from build123d import *

# Parameters (mm, degrees)
SKETCH1_R           = 3
BOSS_EXTRUDE1_DEPTH = 1.59


with BuildPart() as part:
    # Sketch1 → Boss-Extrude1 (new body)
    with BuildSketch(Plane.XY):
        with BuildLine():
            ThreePointArc((-5.900608413, 13.97128969), (-4.905988344, 14.048559559), (-4.072428842, 14.59666381))
            ThreePointArc((-4.072428842, 14.59666381), (3.290759997, 15.306914867), (4.701099283, 8.045238095))
            ThreePointArc((4.701099283, 8.045238095), (3.974825904, 5.45), (4.701099283, 2.854761905))
            ThreePointArc((4.701099283, 2.854761905), (0, -5.5), (-4.701099283, 2.854761905))
            ThreePointArc((-4.701099283, 2.854761905), (-3.974825904, 5.45), (-4.701099283, 8.045238095))
            ThreePointArc((-4.701099283, 8.045238095), (-4.911398404, 8.424486778), (-5.091164818, 8.819124992))
            ThreePointArc((-5.091164818, 8.819124992), (-5.686991836, 9.619268653), (-6.595201124, 10.032058678))
            Line((-6.595201124, 10.032058678), (-25.459894057, 13.358413024))
            Line((-25.459894057, 13.358413024), (-24.765301346, 17.297644037))
            Line((-24.765301346, 17.297644037), (-5.900608413, 13.97128969))
        make_face()
        Circle(SKETCH1_R, mode=Mode.SUBTRACT)
        with Locations((0, 10.9)):
            Circle(SKETCH1_R, mode=Mode.SUBTRACT)
    extrude(amount=BOSS_EXTRUDE1_DEPTH)


solid = part.part
Here's how the part is built. I have some questions about the finished solid (model axes, mm). A direction names the side the tool comes from. Coordinates: 2 decimals unless noted, no trailing zeros. Order: outer loops, then holes, each group sorted by start corner. A loop starts at its lowest first (then second) coordinate and runs counter-clockwise, first axis right, second up. Notation, with made-up numbers: M 36.25,-5 L 69.25,-5 A34 cw 69.25,32 Z; hole C -29,0 d7. An arc over 180 degrees is marked long. Answer as CSV lines item,"result".
Item 1: Imagine slicing it at C-C on z = 0.7. Write out the boundary of the cut face in (x, y).
Results found:
outline,"M -25.46,13.36 L -6.6,10.03 A2 cw -5.09,8.82 A5.5 ccw -4.7,8.05 A5 cw -4.7,2.85 A5.5 ccw long 4.7,2.85 A5 cw 4.7,8.05 A5.5 ccw -4.07,14.6 A2 cw -5.9,13.97 L -24.77,17.3 Z; hole C 0,0 d6; hole C 0,10.9 d6"
Item 2: On a 3-axis mill with a long thin cutter (end or side, diameter ignored), from which of +Z, -Z, +X, -X, +Y, -Y can I reach the whole of each face in a straight line? I mean faces 1 (the face through (-25.117, 15.3, 0.784)), 2 (the face through (-15.47, 15.66, 0.78)), 3 (the face through (-5.676, 9.61, 0.784)). Say none if no direction works.
Results found:
face 1,"+Z, -Z, -X, +Y"
face 2,"+Z, -Z, +Y"
face 3,"+Z, -Z, -X"
Item 3: Imagine slicing it at A-A on x = 0. Write out the boundary of the cut face in (y, z).
Results found:
outline,"M -5.5,0 L -3,0 L -3,1.59 L -5.5,1.59 Z; M 3,0 L 7.9,0 L 7.9,1.59 L 3,1.59 Z; M 13.9,0 L 16.4,0 L 16.4,1.59 L 13.9,1.59 Z"
Item 4: Imagine slicing it at D-D on y = 10.9. Write out the boundary of the cut face in (x, z), plus the area to 3 significant figures.
Results found:
outline,"M -11.52,0 L -3,0 L -3,1.59 L -11.52,1.59 Z; M 3,0 L 5.5,0 L 5.5,1.59 L 3,1.59 Z"
area,"17.5 mm2"
Item 5: Imagine slicing it at B-B on y = 0. Write out the boundary of the cut face in (x, z), plus the area to 3 significant figures.
Results found:
outline,"M -5.5,0 L -3,0 L -3,1.59 L -5.5,1.59 Z; M 3,0 L 5.5,0 L 5.5,1.59 L 3,1.59 Z"
area,"7.95 mm2"
Item 6: We'd pull the mould along X, two halves only. Please class faces 4 (the face through (0.163, -5.498, 0.784)), 5 (the face through (-4, 8, 0)), 6 (the face through (3.199, 15.374, 0.784)): +X half, -X half, draft (parallel to the pull), parting line (faces both ways), or undercut.
Results found:
face 4,"parting line"
face 5,"draft"
face 6,"undercut"
Item 7: If I drill on line 1 (Y direction, x = 0, z = 0.5); line 2 (X direction, y = 9.75, z = 1.15); line 3 (Y direction, x = -2.5, z = 1), over which ranges is the centre line in solid material (lowest first)?
Results found:
line 1,"-5.5 to -3, 3 to 7.9, 13.9 to 16.4"
line 2,"-5.87 to -2.77, 2.77 to 5.38"
line 3,"-4.9 to -1.66, 1.66 to 9.24, 12.56 to 15.8"
